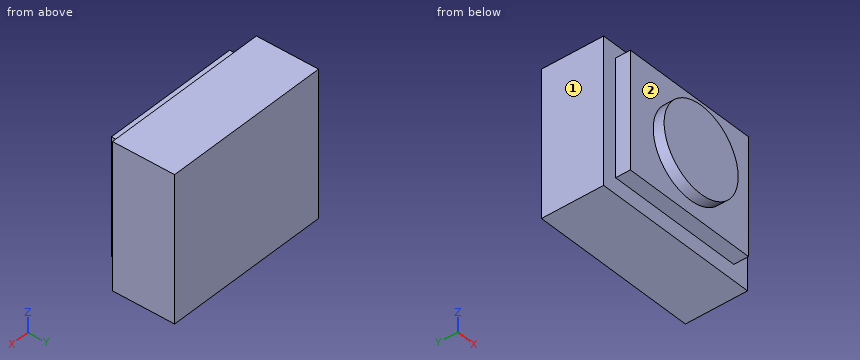
from build123d import *

# Parameters (mm, degrees)
F0_W     = 49.430196
F0_H     = 42.66408
F1_DEPTH = 18.2
F2_W     = 40.59666
F2_H     = 34.206446
F3_DEPTH = 4.3
F4_R     = 12.717394
F5_DEPTH = 3.2


with BuildPart() as f1:
    # F0 (on Front) → F1 (new body)
    with BuildSketch(Plane.XZ):
        Rectangle(F0_W, F0_H)
    extrude(amount=F1_DEPTH)

    # F2 (on face) → F3 (join)
    with BuildSketch(Plane.XZ.offset(18.2)):
        with Locations((-0.281921, 0.469869)):
            Rectangle(F2_W, F2_H)
    extrude(amount=F3_DEPTH)

    # F4 (on face) → F5 (join)
    with BuildSketch(Plane.XZ.offset(22.5)):
        Circle(F4_R)
    extrude(amount=F5_DEPTH)


solid = f1.part
Build history of the part. All positions in model axes, mm. Face numbers are marked on the shaded views. A direction names the side the tool comes from. Give positions to 0.01 mm unless a question says otherwise; leave off trailing zeros. Write each loop counter-clockwise with the first axis right and the second up, starting at its lowest first coordinate (ties: lowest second). Pieces come first, ordered by that corner, then holes. Notation, with made-up numbers: (-35.5, 10.25) - (-5.5, 10.25) arc R32 cw to (-5.5, 47.25) - close; hole circle Ø8 at (13, -1). An arc over 180 degrees is marked (long way). Use one line per item in the form item = value. Start each with the question number.
1. 3-axis set-ups, long thin cutter, end or side, ignore diameter. For the marked faces 1 and 2: which of +Z, -Z, +X, -X, +Y, -Y reach the whole face in a straight line?
2. Drop flat-ended pins along their axis: pin 1 Ø1.3 at (x, y) = (5, -19.5) entering from +Z; pin 2 Ø1 at (x, z) = (18, 6) entering from -Y; pin 3 Ø2 at (y, z) = (-19.5, -5) entering from -X. Give the stop position or say it passes through.
3. Band-saw the part on C-C on z = -16. Write the cut outline in (x, y), plus the area to 3 significant figures.
4. Probe line 1 (Y direction, x = 13.5, z = -9); line 2 (Y direction, x = 5, z = 19); line 3 (Z direction, x = 13.5, y = -20). List the from-to ranges inside material, lowest first. Write a range as [from, to].
5. Band-saw the part on B-B on x = 14.5. Write the cut outline in (y, z), plus the area to 3 significant figures.
6. Band-saw the part on D-D on x = 0. Write the cut outline in (y, z), plus the area to 3 significant figures.
7. Band-saw the part on A-A on z = 0. Write the cut outline in (x, y), plus the area to 3 significant figures.
Conclusion:
q1.face_1 = +Z, -Z, -X, +Y, -Y
q1.face_2 = -Y
q2.pin_1 = 17.57
q2.pin_2 = -22.5
q2.pin_3 = -20.58
q3.outline = (-24.72, -18.2) - (-20.58, -18.2) - (-20.58, -22.5) - (20.02, -22.5) - (20.02, -18.2) - (24.72, -18.2) - (24.72, 0) - (-24.72, 0) - close
q3.area = 1,070 mm²
q4.line_1 = [-22.5, 0]
q4.line_2 = [-18.2, 0]
q4.line_3 = [-16.63, 17.57]
q5.outline = (-22.5, -16.63) - (-18.2, -16.63) - (-18.2, -21.33) - (0, -21.33) - (0, 21.33) - (-18.2, 21.33) - (-18.2, 17.57) - (-22.5, 17.57) - close
q5.area = 924 mm²
q6.outline = (-25.7, -12.72) - (-22.5, -12.72) - (-22.5, -16.63) - (-18.2, -16.63) - (-18.2, -21.33) - (0, -21.33) - (0, 21.33) - (-18.2, 21.33) - (-18.2, 17.57) - (-22.5, 17.57) - (-22.5, 12.72) - (-25.7, 12.72) - close
q6.area = 1,000 mm²
q7.outline = (-24.72, -18.2) - (-20.58, -18.2) - (-20.58, -22.5) - (-12.72, -22.5) - (-12.72, -25.7) - (12.72, -25.7) - (12.72, -22.5) - (20.02, -22.5) - (20.02, -18.2) - (24.72, -18.2) - (24.72, 0) - (-24.72, 0) - close
q7.area = 1,160 mm²
